Can you work these out from the model? Positions are in its coordinate system, mm. Face numbers are marked on the shaded views. Give positions to 0.01 mm unless a question says otherwise; leave off trailing zeros. Loops run counter-clockwise (first coordinate to the right, second up) from the corner with the lowest first, then second, coordinate; pieces in that order, holes last. Notation, with made-up numbers: M -7.5,-1.5 L 25.5,-1.5 A10 ccw 25.5,12.5 Z; hole C -3.5,59.25 d2. An arc over 180 degrees is marked long. Answer as a JSON object with one key per item and string values.
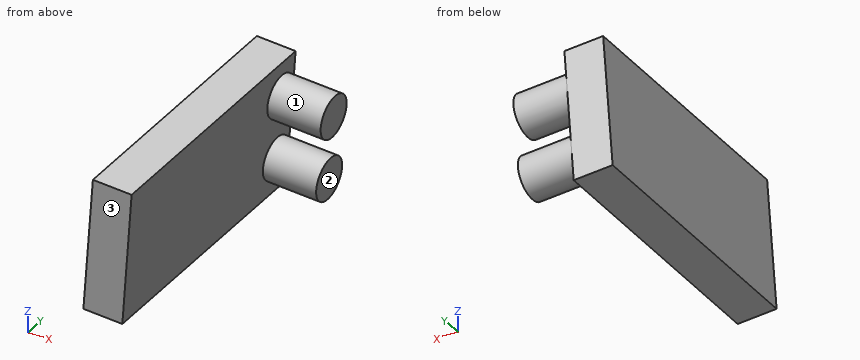
```python
from build123d import *

# Parameters (mm, degrees)
BOSS_EXTRUDE1_DEPTH = 25.4
BOSS_EXTRUDE2_DEPTH = 25.4
SKETCH3_R           = 2
BOSS_EXTRUDE3_DEPTH = 5


with BuildPart() as part:
    # Sketch1 → Boss-Extrude1 (new body)
    with BuildSketch(Plane(origin=(0, 0, 0), x_dir=(1, 0, 0), z_dir=(0, 1, 0))):
        Polygon((83.176569024, -44.663089882), (25.185203896, -48.709261314), (-35.715075295, 41.609133969), (-10.223479979, 93.854215086), (98.44468436, 101.436206322), (130.944454172, 53.237296637), align=None)
        Polygon((28.400509379, -42.119485598), (-28.400509379, 42.119485598), (-6.124219546, 87.774790999), (95.229378877, 94.846430606), (123.629888256, 52.726945008), (79.07730859, -38.583665795), align=None, mode=Mode.SUBTRACT)
    extrude(amount=BOSS_EXTRUDE1_DEPTH)

    # Sketch2 → Boss-Extrude2 (add)
    with BuildSketch(Plane(origin=(0, 25.4, 0), x_dir=(1, 0, 0), z_dir=(0, 1, 0))):
        Polygon((123.193813482, 58.976945008), (124.063847882, 46.507260162), (131.411983768, 47.019954034), (130.541949367, 59.489638879), align=None)
    extrude(amount=-BOSS_EXTRUDE2_DEPTH)

    # Sketch3 → Boss-Extrude3 (add)
    with BuildSketch(Plane(origin=(134.040133914, 0, -9.35224338), x_dir=(-0.06960275203236939, 0, -0.9975747876272337), z_dir=(0.9975747876272337, 0, -0.06960275203236939))):
        with Locations(Location((41.009284939, 23.4, 0), (0, 0, 90))):
            Circle(SKETCH3_R)
        with Locations(Location((47.009284939, 23.4, 0), (0, 0, 180))):
            Circle(SKETCH3_R)
    extrude(amount=BOSS_EXTRUDE3_DEPTH)

    # SurfaceCut1
    split(bisect_by=Plane(origin=(130.455463613, 0, -9.286150729), x_dir=(-0.07100287910742022, 0, -0.9974761105703019), z_dir=(0.9974761105703019, 0, -0.07100287910742022)), keep=Keep.TOP)


solid = part.part
```
1) Will these pins go through, and if not, where does the flat tip stop? pin 1 Ø6 at (y, z) = (10.5, -53) entering from +X; pin 2 Ø3 at (y, z) = (5.5, -49.5) entering from +X.
Answer list:
{"pin 1": "x = 131.2", "pin 2": "x = 131.34"}
2) Suppose I cut it at B-B, the plane x = 128.75. Write out the boundary of the cut face in (y, z), and give its area (3 significant figures).
Answer list:
{"outline": "M 0,-59.36 L 25.4,-59.36 L 25.4,-46.83 L 0,-46.83 Z", "area": "318 mm^2"}
3) Suppose I cut it at A-A, the plane y = 22.75. Write out the boundary of the cut face in (x, z), and give its area (3 significant figures).
Answer list:
{"outline": "M 126.9,-59.24 L 130.54,-59.49 L 130.64,-58.13 L 135.62,-58.48 L 135.89,-54.71 L 130.9,-54.36 L 131.05,-52.15 L 136.04,-52.5 L 136.31,-48.72 L 131.32,-48.38 L 131.41,-47.02 L 127.79,-46.77 Z", "area": "83.4 mm^2"}
4) Please list where these lines run through material, in increasing order: line 1 along X through (y, z) = (11.25, -51); line 2 along Y through (x, z) = (132, -55.5); line 3 along X through (y, z) = (18.75, -47.5). Write a range as from..to.
Answer list:
{"line 1": "127.49..131.13", "line 2": "21.58..25.22", "line 3": "127.74..131.38"}
5) If we mould it in two halves opening along X, with no side actions, what happens to the marked faces 1, 2 and 3? For each: +X half, -X half, draft (parallel to the pull), parting line (faces both ways), or undercut.
Answer list:
{"face 1": "undercut", "face 2": "+X half", "face 3": "draft"}
6) Suppose I cut it at C-C, the plane y = 15. Write out the boundary of the cut face in (x, z).
Answer list:
{"outline": "M 126.9,-59.24 L 130.54,-59.49 L 131.41,-47.02 L 127.79,-46.77 Z"}
